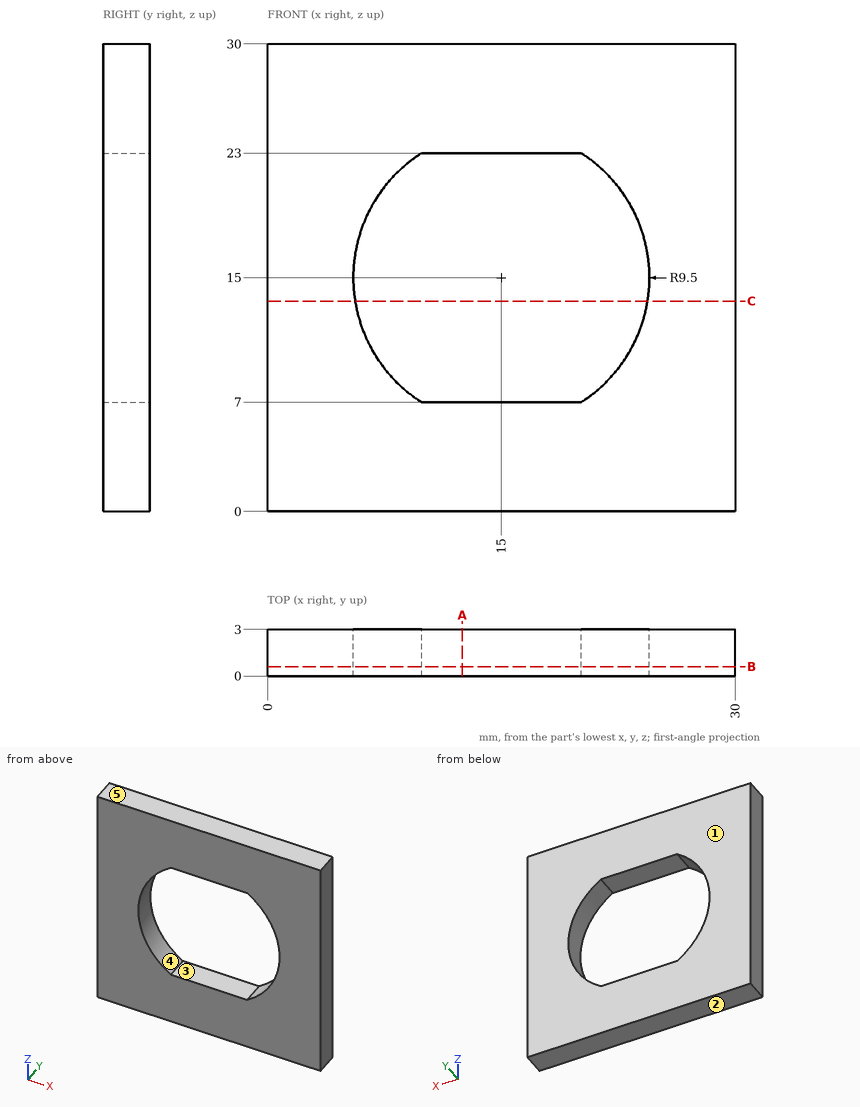
Geometry check sheet. Reference: drawing and pictorial views, mm from the part's lowest x, y, z. A direction names the side the tool comes from. Coordinates: 2 decimals unless noted, no trailing zeros. Order: outer loops, then holes, each group sorted by start corner. A loop starts at its lowest first (then second) coordinate and runs counter-clockwise, first axis right, second up. Notation, with made-up numbers: (-13, -9) -> (45, -9) arc R30 ccw to (45, 28) -> close; hole circle Ø9 at (-27, -23). An arc over 180 degrees is marked (long way). Put each result on its own line as item: value. Start each with the question number.
1) Cross-section at B-B (y = 0.6). Enter the section's corners in (x, z).
2) Material ranges on L1, parallel to Z at x = 23, y = 2.8; L2, parallel to Z at x = 13.5, y = 0.6; L3, parallel to X at y = 0.75, z = 21.75, recorded low to high.
3) Cross-section at C-C (z = 13.5). Enter the section's corners in (x, y).
4) Tool access check on the marked faces 4 and 5. Record the directions out of +Z, -Z, +X, -X, +Y, -Y that give a thin tool (end or side, any length) a straight path to the whole face; none if there is none.
5) Cross-section at A-A (x = 12.5). Enter the section's corners in (y, z).
6) Release check for a two-part mould opening along Z. For the marked faces 1, 2 and 3 record: pulls with the +Z half, pulls with the -Z half, needs draft (parallel to the pull), parting line crosses it, or undercut.
Geometry check:
1. outline: (0, 0) -> (30, 0) -> (30, 30) -> (0, 30) -> close; hole (9.88, 7) -> (20.12, 7) arc R9.5 ccw to (20.12, 23) -> (9.88, 23) arc R9.5 ccw to start
2. L1: z = 0 to 9.88, 20.12 to 30
2. L2: z = 0 to 7, 23 to 30
2. L3: x = 0 to 8.32, 21.68 to 30
3. outline: (0, 0) -> (5.62, 0) -> (5.62, 3) -> (0, 3) -> close; (24.38, 0) -> (30, 0) -> (30, 3) -> (24.38, 3) -> close
4. face 4: +Y, -Y
4. face 5: +Z, +X, -X, +Y, -Y
5. outline: (0, 0) -> (3, 0) -> (3, 7) -> (0, 7) -> close; (0, 23) -> (3, 23) -> (3, 30) -> (0, 30) -> close
6. face 1: needs draft
6. face 2: pulls with the -Z half
6. face 3: undercut
